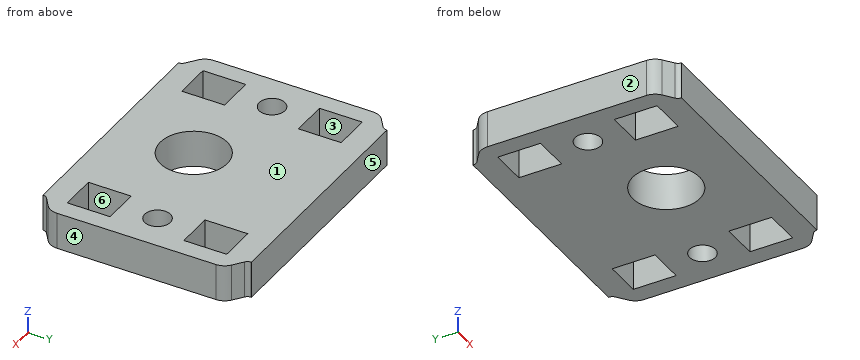
from build123d import *

# Parameters (mm, degrees)
SKETCH_1_W           = 38.55
SKETCH_1_H           = 34.06926437
EXTRUDE_1_DEPTH      = 6
SKETCH_2_R           = 5.475
CUT_EXTRUDE_1_DEPTH  = 7
EXTRUDE_2_DEPTH      = 6
SKETCH_3_R           = 2.1
SKETCH_3_W           = 7
SKETCH_3_H           = 6
CUT_EXTRUDE_13_DEPTH = 7
EXTRUDE_21_DEPTH     = 6
SKETCH_31_R          = 2.1
SKETCH_31_W          = 7
SKETCH_31_H          = 6
CUT_EXTRUDE_14_DEPTH = 7


with BuildPart() as part:
    # Эскиз1 → Бобышка-Вытянуть1 (new body)
    with BuildSketch(Plane.XY):
        with Locations((4.02043073, 23.206158468)):
            Rectangle(SKETCH_1_W, SKETCH_1_H)
    extrude(amount=EXTRUDE_1_DEPTH)

    # Эскиз2 → Вырез-Вытянуть1 (cut, through all)
    with BuildSketch(Plane.XY.offset(6)):
        with Locations((3.40043073, 19.378379342)):
            Circle(SKETCH_2_R)
    extrude(amount=-CUT_EXTRUDE_1_DEPTH, mode=Mode.SUBTRACT)

    # Эскиз23 → Бобышка-Вытянуть2 (add)
    with BuildSketch(Plane(origin=(-26.70456927, 23.171526283, 6), x_dir=(0, 1, 0), z_dir=(0, 0, -1))):
        with BuildLine():
            Line((13, 53), (-13, 53))
            ThreePointArc((-13, 53), (-14.118033989, 52.736067977), (-15, 52))
            Line((-15, 52), (-16.2, 50.4))
            ThreePointArc((-16.2, 50.4), (-16.552786405, 50.105572809), (-17, 50))
            Line((-17, 50), (17, 50))
            ThreePointArc((17, 50), (16.552786405, 50.105572809), (16.2, 50.4))
            Line((16.2, 50.4), (15, 52))
            ThreePointArc((15, 52), (14.118033989, 52.736067977), (13, 53))
        make_face()
    extrude(amount=EXTRUDE_2_DEPTH)

    # Эскиз3 → Вырез-Вытянуть13 (cut, through all)
    with BuildSketch(Plane(origin=(-26.70456927, 23.171526283, 0), x_dir=(0, 1, 0), z_dir=(0, 0, -1))):
        with Locations((0, 47)):
            Circle(SKETCH_3_R)
        with Locations((9.531849908, 47)):
            Rectangle(SKETCH_3_W, SKETCH_3_H)
        with Locations((-9.531849908, 47)):
            Rectangle(SKETCH_3_W, SKETCH_3_H)
    extrude(amount=-CUT_EXTRUDE_13_DEPTH, mode=Mode.SUBTRACT)

    # Эскиз24 → Бобышка-Вытянуть21 (add)
    with BuildSketch(Plane(origin=(34.74543073, 23.171526283, 6), x_dir=(0, -1, 0), z_dir=(0, 0, -1))):
        with BuildLine():
            Line((13, 53), (-13, 53))
            ThreePointArc((-13, 53), (-14.118033989, 52.736067977), (-15, 52))
            Line((-15, 52), (-16.2, 50.4))
            ThreePointArc((-16.2, 50.4), (-16.552786405, 50.105572809), (-17, 50))
            Line((-17, 50), (17, 50))
            ThreePointArc((17, 50), (16.552786405, 50.105572809), (16.2, 50.4))
            Line((16.2, 50.4), (15, 52))
            ThreePointArc((15, 52), (14.118033989, 52.736067977), (13, 53))
        make_face()
    extrude(amount=EXTRUDE_21_DEPTH)

    # Эскиз31 → Вырез-Вытянуть14 (cut, through all)
    with BuildSketch(Plane(origin=(34.74543073, 23.171526283, 0), x_dir=(0, -1, 0), z_dir=(0, 0, -1))):
        with Locations((0, 47)):
            Circle(SKETCH_31_R)
        with Locations((9.531849908, 47)):
            Rectangle(SKETCH_31_W, SKETCH_31_H)
        with Locations((-9.531849908, 47)):
            Rectangle(SKETCH_31_W, SKETCH_31_H)
    extrude(amount=-CUT_EXTRUDE_14_DEPTH, mode=Mode.SUBTRACT)


solid = part.part
Build history of the part. All positions in model axes, mm. Face numbers are marked on the shaded views. A direction names the side the tool comes from. Round coordinates to 2 decimals unless told otherwise and drop trailing zeros. Loops run counter-clockwise (first coordinate to the right, second up) from the corner with the lowest first, then second, coordinate; pieces in that order, holes last. Notation, with made-up numbers: (-16.5, 7) -> (25.5, 7) arc R34 cw to (25.5, 43) -> close; hole circle Ø10 at (-2, -25). An arc over 180 degrees is marked (long way). One line per item, written item: value. Start each with the question number.
Q1. Cut at B-B on x = 4. List the corners of the cut face in (y, z), plus the area to 3 significant figures.
Q2. Two-plate mould, pull along X, no slides. Class the marked faces 1, 2, 3 and 4: released by +X, released by -X, zero draft, split by the parting line, or undercut.
Q3. Cut at A-A on y = 11. List the corners of the cut face in (x, z), plus the area to 3 significant figures.
Q4. 3-axis set-ups, long thin cutter, end or side, ignore diameter. For the marked faces 5 and 6: which of +Z, -Z, +X, -X, +Y, -Y reach the whole face in a straight line?
Q5. Probe line 1 along X through (y, z) = (31.5, 4.2); line 2 along Y through (x, z) = (21, 1.1); line 3 along X through (y, z) = (15, 0.6). List the from-to ranges inside material, lowest first.
Q6. Cut at C-C on x = 21.5. List the corners of the cut face in (y, z), plus the area to 3 significant figures.
Q7. Drop a flat-ended pin along its axis: pin 1 Ø5.5 at (x, y) = (-12.25, 23.17) entering from -Z. Give the stop position or say it passes through.
Q8. Cut at D-D on z = 4.4. Count the separate pieces of the cut face and the enclosed holes in it, plus the area to 3 significant figures.
Computed:
1. outline: (6.17, 0) -> (13.94, 0) -> (13.94, 6) -> (6.17, 6) -> close; (24.82, 0) -> (40.24, 0) -> (40.24, 6) -> (24.82, 6) -> close
1. area: 139 mm²
2. face 1: zero draft
2. face 2: released by -X
2. face 3: undercut
2. face 4: released by +X
3. outline: (-18.25, 0) -> (-15.25, 0) -> (-15.25, 6) -> (-18.25, 6) -> close; (-9.25, 0) -> (17.3, 0) -> (17.3, 6) -> (-9.25, 6) -> close; (23.3, 0) -> (26.3, 0) -> (26.3, 6) -> (23.3, 6) -> close
3. area: 195 mm²
4. face 5: +Z, -Z, +X, -X, +Y
4. face 6: +Z, -Z
5. line 1: -18.25 to -15.25, -9.25 to 17.3, 23.3 to 26.3
5. line 2: 6.17 to 10.14, 17.14 to 21.19, 25.15 to 29.2, 36.2 to 40.24
5. line 3: -18.25 to -15.25, -9.25 to 0.11, 6.69 to 17.3, 23.3 to 26.3
6. outline: (6.17, 0) -> (10.14, 0) -> (10.14, 6) -> (6.17, 6) -> close; (17.14, 0) -> (21.45, 0) -> (21.45, 6) -> (17.14, 6) -> close; (24.89, 0) -> (29.2, 0) -> (29.2, 6) -> (24.89, 6) -> close; (36.2, 0) -> (40.24, 0) -> (40.24, 6) -> (36.2, 6) -> close
6. area: 99.8 mm²
7. pin 1: z = 0
8. separate pieces: 1
8. enclosed holes: 7
8. area: 1,210 mm²
